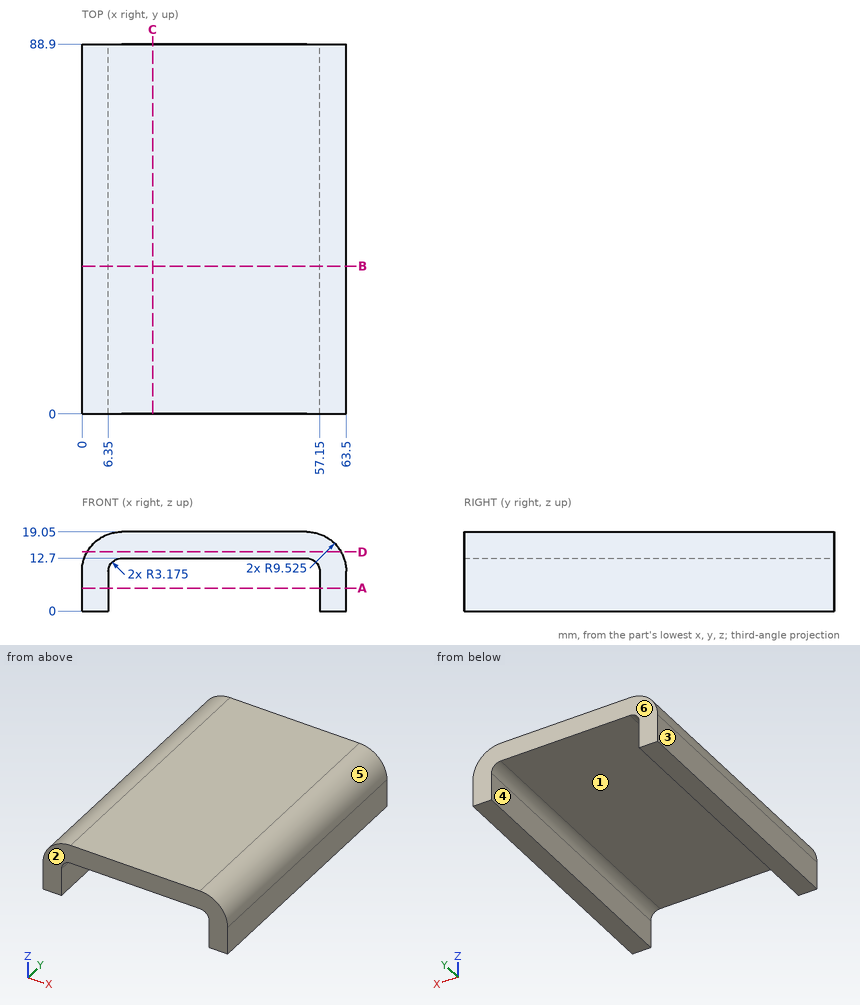
Verification items for this drawing (mm, ordinates from the low corner). A direction names the side the tool comes from. Coordinates: 2 decimals unless noted, no trailing zeros. Write each loop counter-clockwise with the first axis right and the second up, starting at its lowest first coordinate (ties: lowest second). Pieces come first, ordered by that corner, then holes. Notation, with made-up numbers: (-33, 77) -> (-14, 77) arc R22 cw to (-14, 104) -> close; hole circle Ø7 at (-23.75, 24.25). An arc over 180 degrees is marked (long way). One line per item, written item: value. Start each with the question number.
Q1. Access from +Z, -Z, +X, -X, +Y, -Y to the whole of each face (thin tool, end or side, straight path). Record for the marked faces 1 and 2.
Q2. Cross-section at D-D on z = 14.25. Enter the section's corners in (x, y), and give its area (3 significant figures).
Q3. Cross-section at B-B on y = 35.5. Enter the section's corners in (x, z) (3 decimals), and give its area (3 significant figures).
Q4. Mould release check, pull along X, two halves, no side actions. Record for the marked faces 3, 4, 5 and 6: pulls with the +X half, pulls with the -X half, needs draft (parallel to the pull), parting line crosses it, or undercut.
Q5. Cross-section at C-C on x = 17. Enter the section's corners in (y, z), and give its area (3 significant figures).
Q6. Cross-section at A-A on z = 5.5. Enter the section's corners in (x, y), and give its area (3 significant figures).
Q7. Thickness scan on L1, parallel to X at y = 72, z = 5.5; L2, parallel to Z at x = 53, y = 79.5; L3, parallel to X at y = 81, z = 11.25. Record the ranges inside material, lowest first. Write a range as from..to.
Q8. Go/stop test with a flat-tipped pin: P1, Ø22, axis at x = 34, y = 40.5, coming from the -Z side. Record where the tip stops, or that it passes through.
Checked values:
1. face 1: -Z, +Y, -Y
1. face 2: +Z, -Z, +X, -X, -Y
2. outline: (1.25, 0) -> (62.25, 0) -> (62.25, 88.9) -> (1.25, 88.9) -> close
2. area: 5,420 mm²
3. outline: (0, 0) -> (6.35, 0) -> (6.35, 9.525) arc R3.175 cw to (9.525, 12.7) -> (53.975, 12.7) arc R3.175 cw to (57.15, 9.525) -> (57.15, 0) -> (63.5, 0) -> (63.5, 9.525) arc R9.525 ccw to (53.975, 19.05) -> (9.525, 19.05) arc R9.525 ccw to (0, 9.525) -> close
3. area: 530 mm²
4. face 3: pulls with the -X half
4. face 4: undercut
4. face 5: pulls with the +X half
4. face 6: needs draft
5. outline: (0, 12.7) -> (88.9, 12.7) -> (88.9, 19.05) -> (0, 19.05) -> close
5. area: 565 mm²
6. outline: (0, 0) -> (6.35, 0) -> (6.35, 88.9) -> (0, 88.9) -> close; (57.15, 0) -> (63.5, 0) -> (63.5, 88.9) -> (57.15, 88.9) -> close
6. area: 1,130 mm²
7. L1: x = 0..6.35, 57.15..63.5
7. L2: z = 12.7..19.05
7. L3: x = 0.16..6.86, 56.64..63.34
8. P1: stops at z = 12.7
